Drawing for the job (mm, zero at the part's lowest x, y, z). Round coordinates to 2 decimals unless told otherwise and drop trailing zeros. Order: outer loops, then holes, each group sorted by start corner. A loop starts at its lowest first (then second) coordinate and runs counter-clockwise, first axis right, second up. Notation, with made-up numbers: M 4,-38.5 L 16,-38.5 A8 ccw 16,-32.5 Z; hole C 54,48 d11. An arc over 180 degrees is marked long. One line per item, written item: value. Start each with the question number.
Item 1: Pin check, flat tip, straight feed: pin 1 (1.5 mm diameter, centred on x = 11, y = 17.5, fed in from -Z). Stop position of the tip, or through.
Item 2: Probe L1, parallel to Y at x = 8, z = 3.1; L2, parallel to Y at x = 6, z = 1; L3, parallel to X at y = 11, z = 4.1. List the from-to ranges inside material, lowest first.
Item 3: Band-saw the part on A-A, the plane y = 33. Write the cut outline in (x, z).
Item 4: Band-saw the part on C-C, the plane x = 14.75. Write the cut outline in (y, z).
Item 5: Band-saw the part on B-B, the plane z = 0.9. Give the number of separate pieces and of enclosed holes in the cut face, then the cut area to 3 significant figures.
Item 6: Two-plate mould, pull along Y, no slides. Class the marked faces 1, 2 and 3: +Y half, -Y half, draft (parallel to the pull), parting line (faces both ways), or undercut.
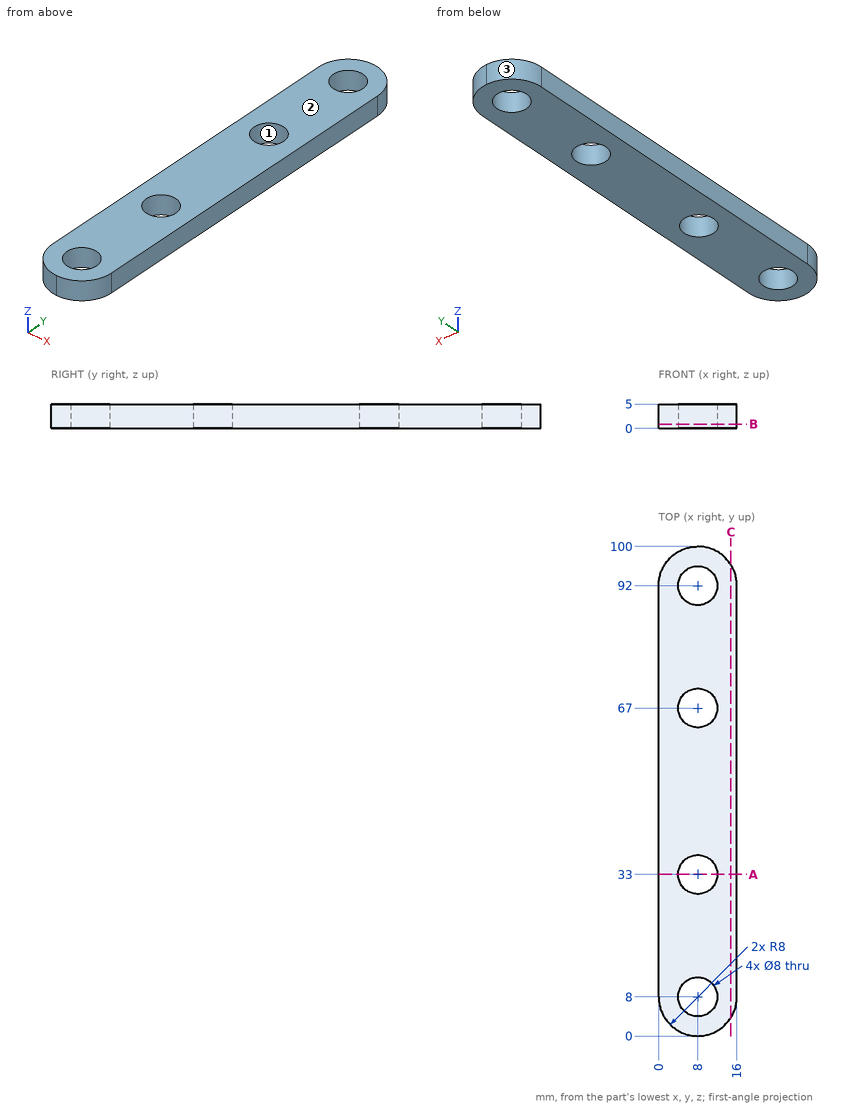
Output:
1. pin 1: stops at z = 0
2. L1: y = 0 to 4, 12 to 29, 37 to 63, 71 to 88, 96 to 100
2. L2: y = 0.25 to 4.54, 11.46 to 29.54, 36.46 to 63.54, 70.46 to 88.54, 95.46 to 99.75
2. L3: x = 0 to 5.35, 10.65 to 16
3. outline: M 0,0 L 4,0 L 4,5 L 0,5 Z; M 12,0 L 16,0 L 16,5 L 12,5 Z
4. outline: M 3.71,0 L 96.29,0 L 96.29,5 L 3.71,5 Z
5. separate pieces: 1
5. enclosed holes: 4
5. area: 1,340 mm²
6. face 1: undercut
6. face 2: draft
6. face 3: +Y half
